Design review of the part built by this model. Coordinates are the model's own, in mm. Round coordinates to 2 decimals unless told otherwise and drop trailing zeros. Order: outer loops, then holes, each group sorted by start corner. A loop starts at its lowest first (then second) coordinate and runs counter-clockwise, first axis right, second up. Notation, with made-up numbers: M 45.25,-32 L 55.25,-32 A14 cw 55.25,-21 Z; hole C 55,82.25 d11. An arc over 180 degrees is marked long. Use a Markdown table: item, result. Add a question column.
(1) Take a section at D-D (y = 3.25). Count the separate pieces of the cut face and the enclosed holes in it, then the cut area to 3 significant figures.
(2) The part is to be moulded in two halves that separate along Z. For faces 1 (the face through (-21, 4, 50)), 2 (the face through (-101.185, 4.056, 22.819)), 3 (the face through (-21, 8, -1)), 4 (the face through (-21, 4, -50)), say which applies: released by +Z, released by -Z, zero draft, split by the parting line, or undercut.
(3) Take a section at C-C (z = -23.57). Write out the cut boundary in (x, y).
(4) Take a section at A-A (x = -103.57). Write out the cut boundary in (y, z), then the cut area to 3 significant figures.
(5) To check wall thickness, follow probe 1 along X at (y, z) = (4.75, -23.57); probe 2 along Z at (x, y) = (-103.57, 2.25); probe 3 along X at (y, z) = (7.5, -0.5). State the ranges of each line that lie inside material, in increasing order. Write a range as from..to.
(6) Take a section at B-B (x = -80). Write out the cut boundary in (y, z), then the cut area to 3 significant figures.
```python
from build123d import *

# Parameters (mm, degrees)
SKETCH1_W           = 250
SKETCH1_H           = 100
BOSS_EXTRUDE1_DEPTH = 8
SKETCH2_R           = 2.5
CUT_EXTRUDE1_DEPTH  = 8
SKETCH3_R           = 3
CUT_EXTRUDE2_DEPTH  = 8
SKETCH5_W           = 40
SKETCH5_H           = 100
CUT_EXTRUDE3_DEPTH  = 10
SKETCH6_R           = 20
CUT_EXTRUDE4_DEPTH  = 8


with BuildPart() as part:
    # Sketch1 → Boss-Extrude1 (new body)
    with BuildSketch(Plane(origin=(0, 0, 0), x_dir=(1, 0, 0), z_dir=(0, 1, 0))):
        Rectangle(SKETCH1_W, SKETCH1_H)
    extrude(amount=BOSS_EXTRUDE1_DEPTH)

    # Sketch2 → Cut-Extrude1 (cut)
    with BuildSketch(Plane(origin=(0, 8, 0), x_dir=(1, 0, 0), z_dir=(0, 1, 0))):
        with Locations((-103.57, 23.57)):
            Circle(SKETCH2_R)
        with Locations((-56.43, 23.57)):
            Circle(SKETCH2_R)
        with Locations((-56.43, -23.57)):
            Circle(SKETCH2_R)
        with Locations((-103.57, -23.57)):
            Circle(SKETCH2_R)
    extrude(amount=-CUT_EXTRUDE1_DEPTH, mode=Mode.SUBTRACT)

    # Sketch3 → Cut-Extrude2 (cut)
    with BuildSketch(Plane(origin=(0, 8, 0), x_dir=(1, 0, 0), z_dir=(0, 1, 0))):
        with Locations((-80, 23.57)):
            Circle(SKETCH3_R)
        with Locations((-103.57, 0)):
            Circle(SKETCH3_R)
        with Locations((-80, -23.57)):
            Circle(SKETCH3_R)
    extrude(amount=-CUT_EXTRUDE2_DEPTH, mode=Mode.SUBTRACT)

    # Sketch5 → Cut-Extrude3 (cut)
    with BuildSketch(Plane.XZ):
        with Locations((105, 0)):
            Rectangle(SKETCH5_W, SKETCH5_H)
    extrude(amount=-CUT_EXTRUDE3_DEPTH, mode=Mode.SUBTRACT)

    # Sketch6 → Cut-Extrude4 (cut)
    with BuildSketch(Plane.XZ):
        with Locations((40, 0)):
            Circle(SKETCH6_R)
    extrude(amount=-CUT_EXTRUDE4_DEPTH, mode=Mode.SUBTRACT)


solid = part.part
```
Verdict:
| question | item | result |
|---|---|---|
| 1 | separate pieces | 1 |
| 1 | enclosed holes | 8 |
| 1 | area | 19,600 mm^2 |
| 2 | face 1 | released by +Z |
| 2 | face 2 | undercut |
| 2 | face 3 | zero draft |
| 2 | face 4 | released by -Z |
| 3 | outline | M -125,0 L -106.07,0 L -106.07,8 L -125,8 Z; M -101.07,0 L -83,0 L -83,8 L -101.07,8 Z; M -77,0 L -58.93,0 L -58.93,8 L -77,8 Z; M -53.93,0 L 85,0 L 85,8 L -53.93,8 Z |
| 4 | outline | M 0,-50 L 8,-50 L 8,-26.07 L 0,-26.07 Z; M 0,-21.07 L 8,-21.07 L 8,-3 L 0,-3 Z; M 0,3 L 8,3 L 8,21.07 L 0,21.07 Z; M 0,26.07 L 8,26.07 L 8,50 L 0,50 Z |
| 4 | area | 672 mm^2 |
| 5 | probe 1 | x = -125..-106.07, -101.07..-83, -77..-58.93, -53.93..85 |
| 5 | probe 2 | z = -50..-26.07, -21.07..-3, 3..21.07, 26.07..50 |
| 5 | probe 3 | x = -125..-106.53, -100.61..20.01, 59.99..85 |
| 6 | outline | M 0,-50 L 8,-50 L 8,-26.57 L 0,-26.57 Z; M 0,-20.57 L 8,-20.57 L 8,20.57 L 0,20.57 Z; M 0,26.57 L 8,26.57 L 8,50 L 0,50 Z |
| 6 | area | 704 mm^2 |
